Check sheet for the drawn part. Datum: minimum x, y, z corner. Units: mm. A direction names the side the tool comes from. Round coordinates to 2 decimals unless told otherwise and drop trailing zeros. Write each loop counter-clockwise with the first axis right and the second up, starting at its lowest first coordinate (ties: lowest second). Pieces come first, ordered by that corner, then holes. Notation, with made-up numbers: (41.25, -27) - (74.25, -27) arc R31 cw to (74.25, 4) - close; hole circle Ø10 at (58, 45). An arc over 180 degrees is marked (long way). Answer as a JSON object with one key per item and string values. Group by question number.
Item 1: Thickness scan on line 1 (Y direction, x = 3, z = 51); line 2 (Z direction, x = 4, y = 20) (1 decimal); line 3 (Z direction, x = 9.25, y = 8.75) (1 decimal). Record the ranges inside material, lowest first.
Item 2: Sectioned sample at B-B on x = 6.5. Count the separate pieces of the cut face and the enclosed holes in it, plus the area to 3 significant figures.
Item 3: Sectioned sample at C-C on z = 71.5. Record the boundary of the cut face in (x, y), plus the area to 3 significant figures.
Item 4: Gauge pin test, flat ends, axial feed: P1, Ø1.5, axis at x = 2, y = 3, coming from the +Z side; P2, Ø4, axis at x = 2, y = 23, coming from the +Z side; P3, Ø5, axis at x = 7.5, y = 4, coming from the +Z side (1 decimal); P4, Ø1.5, axis at x = 4, y = 9.5, coming from the -Z side. Record the tip position at first contact, or that the pin passes through.
Item 5: Sectioned sample at A-A on y = 7.5. Record the boundary of the cut face in (x, z) (1 decimal).
Item 6: Sectioned sample at D-D on y = 13.5. Record the boundary of the cut face in (x, z).
Item 7: Set-up check for the marked faces 1 and 2: record each of +Z, -Z, +X, -X, +Y, -Y from which the full face is reachable in a straight line by a thin tool's end or side.
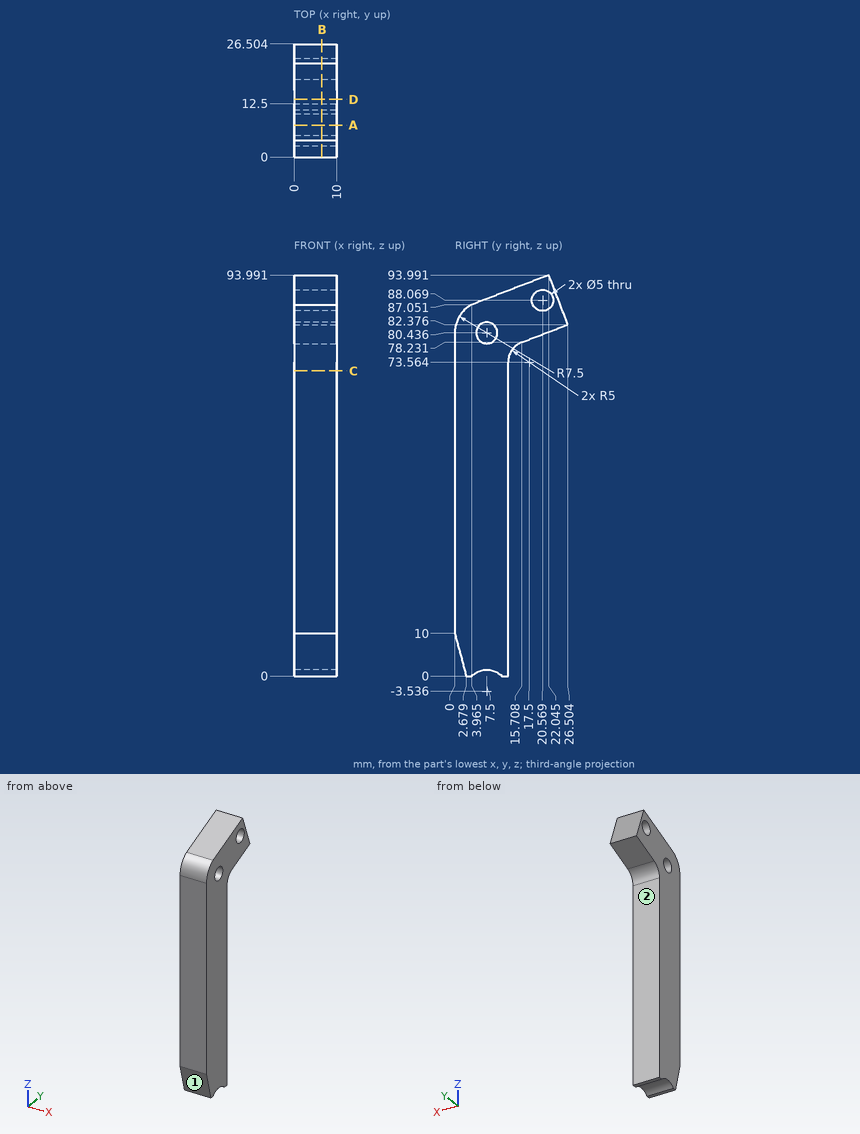
Completed:
{
 "1": {"line 1": "0 to 12.5", "line 2": "79.9 to 85.6, 90.5 to 93.2", "line 3": "1.3 to 78.3, 82.6 to 88.9"},
 "2": {"separate pieces": "1", "enclosed holes": "2", "area": "1,190 mm²"},
 "3": {"outline": "(0, 0) - (10, 0) - (10, 12.5) - (0, 12.5) - close", "area": "125 mm²"},
 "4": {"P1": "z = 86.93", "P2": "z = 93.99", "P3": "z = 88", "P4": "z = 0.64"},
 "5": {"outline": "(0, 1.5) - (10, 1.5) - (10, 77.9) - (0, 77.9) - close; (0, 82.9) - (10, 82.9) - (10, 88.4) - (0, 88.4) - close"},
 "6": {"outline": "(0, 76.56) - (10, 76.56) - (10, 90.71) - (0, 90.71) - close"},
 "7": {"face 1": "-Z, +X, -X, -Y", "face 2": "-Z, +X, -X, +Y"}
}
